Verification items for the finished model (mm, model axes). A direction names the side the tool comes from. Give positions to 0.01 mm unless a question says otherwise; leave off trailing zeros. Loops run counter-clockwise (first coordinate to the right, second up) from the corner with the lowest first, then second, coordinate; pieces in that order, holes last. Notation, with made-up numbers: (19.5, -31.5) - (77.5, -31.5) arc R24 ccw to (77.5, 6.5) - close; hole circle Ø9 at (-32.75, 42). An arc over 180 degrees is marked (long way). One line per item, written item: value. Start each with the question number.
1. Gauge pin test, flat ends, axial feed: pin 1 (10 mm diameter, centred on x = -31, y = 6, fed in from +Z); pin 2 (12 mm diameter, centred on x = -7.5, z = -14.5, fed in from -Y). Record the tip position at first contact, or that the pin passes through.
2. Sectioned sample at C-C (z = -19.5). Record the cut outline in (x, y), plus the area to 3 significant figures.
3. Mould release check, pull along X, two halves, no side actions. Record for faces 1 (the flat face through (0, 10, -39)), 2 (the flat face through (-20, 20, -37)), 3 (the flat face through (-41, 10, -37)), 4 (the flat face through (-0.991, 9, -37)): pulls with the +X half, pulls with the -X half, needs draft (parallel to the pull), parting line crosses it, or undercut.
4. Access from +Z, -Z, +X, -X, +Y, -Y to the whole of each face (thin tool, end or side, straight path). Record for faces 5 (the flat face through (-20, 10, 0)), 6 (the flat face through (-29, 9, -70.626)).
5. Sectioned sample at B-B (x = -25). Record the cut outline in (y, z), plus the area to 3 significant figures.
6. Scan lines: L1, parallel to X at y = 9.25, z = -53.5; L2, parallel to Z at x = -31, y = 14.75; L3, parallel to Z at x = -10, y = 1.5. Record each from-to range of solid material in increasing order. Write a range as [from, to].
7. Sectioned sample at A-A (y = 14.75). Record the cut outline in (x, z).
Autodesk Inventor part; units mm, degrees
ref_plane "YZ Plane" through (0, 0, 0) normal (1, 0, 0) x (0, 1, 0)
ref_plane "XZ Plane" through (0, 0, 0) normal (0, 1, 0) x (-1, 0, 0)
ref_plane "XY Plane" through (0, 0, 0) normal (0, 0, 1) x (1, 0, 0)
sketch "Эскиз1" plane through (0, 0, 0) normal (0, 1, 0) x (-1, 0, 0)
  line L0 (0, 0) -> (41, 0)
  line L1 (41, 0) -> (41, -76)
  line L2 (41, -76) -> (0, -76)
  line L3 (0, -76) -> (0, 0)
  line L4 (38.493, -5.6262) -> (20.493, -5.6262)
  line L5 (20.493, -5.6262) -> (20.493, -70.6262)
  line L6 (20.493, -70.6262) -> (38.493, -70.6262)
  line L7 (38.493, -70.6262) -> (38.493, -5.6262)
  line L8 (18.991, -5.4252) -> (0.991, -5.4252)
  line L9 (0.991, -5.4252) -> (0.991, -70.4252)
  line L10 (0.991, -70.4252) -> (18.991, -70.4252)
  line L11 (18.991, -70.4252) -> (18.991, -5.4252)
  dimension "d0" = 41
  dimension "d1" = 76
  dimension "d2" = 18
  dimension "d3" = 65
  dimension "d4" = 18
  dimension "d5" = 65
extrude "Выдавливание1" add sketch "Эскиз1" along normal blind 20 contours L0 L1 L2 L3 | L7 L6 L5 L4 | L11 L10 L9 L8
extrude "Выдавливание2" cut sketch "Эскиз1" along normal blind 18 contours L7 L6 L5 L4 | L11 L10 L9 L8
properties part number "Battery_Holder"
Results are:
1. pin 1: stops at z = 0
1. pin 2: stops at y = 18
2. outline: (-41, 0) - (-38.49, 0) - (-38.49, 18) - (-20.49, 18) - (-20.49, 0) - (-18.99, 0) - (-18.99, 18) - (-0.99, 18) - (-0.99, 0) - (0, 0) - (0, 20) - (-41, 20) - close
2. area: 172 mm^2
3. face 1: pulls with the +X half
3. face 2: needs draft
3. face 3: pulls with the -X half
3. face 4: undercut
4. face 5: +Z, +X, -X, +Y, -Y
4. face 6: -Y
5. outline: (0, -76) - (20, -76) - (20, 0) - (0, 0) - (0, -5.63) - (18, -5.63) - (18, -70.63) - (0, -70.63) - close
5. area: 350 mm^2
6. L1: x = [-41, -38.49], [-20.49, -18.99], [-0.99, 0]
6. L2: z = [-76, -70.63], [-5.63, 0]
6. L3: z = [-76, -70.43], [-5.43, 0]
7. outline: (-41, -76) - (0, -76) - (0, 0) - (-41, 0) - close; hole (-38.49, -70.63) - (-20.49, -70.63) - (-20.49, -5.63) - (-38.49, -5.63) - close; hole (-18.99, -70.43) - (-0.99, -70.43) - (-0.99, -5.43) - (-18.99, -5.43) - close
